Read the model definition and answer for the solid it produces. Units are mm, in the model's axes. A direction names the side the tool comes from. Coordinates: 2 decimals unless noted, no trailing zeros. Loops run counter-clockwise (first coordinate to the right, second up) from the corner with the lowest first, then second, coordinate; pieces in that order, holes last.
Q1. Section B-B (z = 3) is taken. Give the vertices of the cut face in (x, y), then the cut area to 3 significant figures.
Q2. Which of the six approach directions +Z, -Z, +X, -X, +Y, -Y give full straight-line access (tool end or side, diameter ignored) to faces 5 (the face through (6.35, 25, 7)), 6 (the face through (12.7, 25, 7)), 7 (the face through (9, 25, 10.16)), 8 (the face through (9, 26, 6.35)), 9 (the face through (-2.974, 5.098, -33.82))?
Q3. Section A-A (y = 33.5) is taken. Give the vertices of the cut face in (x, z).
Q4. Section D-D (z = -41) is taken. Give the vertices of the cut face in (x, y).
Q5. Straight lines are drawn through the part: line 1 (Y direction, x = 4, z = -32.5); line 2 (Y direction, x = -42, z = -5); line 3 (X direction, y = 42.5, z = 5). For each, find the intervals that lie inside material, in ascending order.
Q6. Flat-ended cylindrical pins translate along their axes: P1, Ø5, axis at x = 37.5, z = -27.5, coming from the +Y side; P2, Ø10, axis at y = 19.5, z = 1, coming from the +X side; P3, Ø2, axis at x = -2, y = 4.5, coming from the -Z side; P4, Ø2, axis at y = 40.5, z = -0.11, coming from the -X side. Find the tip coordinate at first contact, or state that the pin passes through.
Q7. The mould has two halves that part along Y. Classify faces 1 (the face through (9, 25, -10.16)), 2 (the face through (9, 26, -6.59)), 3 (the face through (1, 3.81, -32)), 4 (the face through (9, 38.079, 0)): pulls with the +Y half, pulls with the -Y half, needs draft (parallel to the pull), parting line crosses it, or undercut.
Q8. Section C-C (x = -2) is taken. Give the vertices of the cut face in (y, z), then the cut area to 3 significant figures.
from build123d import *

# Parameters (mm, degrees)
SKETCH1_R           = 50.8
BOSS_EXTRUDE1_DEPTH = 6.35
SKETCH2_W           = 6.35
SKETCH2_H           = 20.32
BOSS_EXTRUDE2_DEPTH = 38.1
SKETCH3_R           = 1.1
SKETCH3_W           = 12.939919869
SKETCH3_H           = 22.881654632
CUT_EXTRUDE1_DEPTH  = 12.7
CUT_EXTRUDE2_DEPTH  = 2.54


with BuildPart() as part:
    # Sketch1 → Boss-Extrude1 (new body)
    with BuildSketch(Plane(origin=(0, 0, 0), x_dir=(1, 0, 0), z_dir=(0, 1, 0))):
        Circle(SKETCH1_R)
    extrude(amount=BOSS_EXTRUDE1_DEPTH)

    # Sketch2 → Boss-Extrude2 (add)
    with BuildSketch(Plane(origin=(0, 6.35, 0), x_dir=(1, 0, 0), z_dir=(0, 1, 0))):
        with Locations((9.525, 0)):
            Rectangle(SKETCH2_W, SKETCH2_H)
    extrude(amount=BOSS_EXTRUDE2_DEPTH)

    # Sketch3 → Cut-Extrude1 (cut)
    with BuildSketch(Plane(origin=(6.35, 55.246794414, 64.642959957), x_dir=(0, 0, 1), z_dir=(-1, 0, 0))):
        with Locations((-64.750269074, -14.746794414)):
            Circle(SKETCH3_R)
        with Locations((-64.750269074, -42.546794414)):
            Circle(SKETCH3_R)
        with Locations((-64.762919892, -28.608275818)):
            Rectangle(SKETCH3_W, SKETCH3_H)
    extrude(amount=-CUT_EXTRUDE1_DEPTH, mode=Mode.SUBTRACT)

    # Sketch4 → Cut-Extrude2 (cut)
    with BuildSketch(Plane(origin=(0, 6.35, 0), x_dir=(1, 0, 0), z_dir=(0, 1, 0))):
        Polygon((-7.230978109, 23.634136505), (9.560420722, 23.634136505), (1.164721306, 43.725579037), align=None)
    extrude(amount=-CUT_EXTRUDE2_DEPTH, mode=Mode.SUBTRACT)


solid = part.part
Numbers:
1. outline: (-50.71, 0) - (50.71, 0) - (50.71, 6.35) - (12.7, 6.35) - (12.7, 15.2) - (6.35, 15.2) - (6.35, 6.35) - (-50.71, 6.35) - close; (6.35, 38.08) - (12.7, 38.08) - (12.7, 44.45) - (6.35, 44.45) - close
1. area: 741 mm2
2. face 5: +Z, -Z, -X, +Y
2. face 6: +Z, -Z, +X, +Y
2. face 7: +Z, +X, -X, +Y
2. face 8: +X, -X
2. face 9: +Y
3. outline: (6.35, -10.16) - (12.7, -10.16) - (12.7, -6.59) - (6.35, -6.59) - close; (6.35, 6.35) - (12.7, 6.35) - (12.7, 10.16) - (6.35, 10.16) - close
4. outline: (-29.99, 0) - (29.99, 0) - (29.99, 6.35) - (2.3, 6.35) - (2.3, 3.81) - (0.03, 3.81) - (0.03, 6.35) - (-29.99, 6.35) - close
5. line 1: y = 0 to 3.81
5. line 2: y = 0 to 6.35
5. line 3: x = 6.35 to 12.7
6. P1: stops at y = 6.35
6. P2: stops at x = 12.7
6. P3: stops at z = -50.79
6. P4: passes through
7. face 1: needs draft
7. face 2: undercut
7. face 3: pulls with the +Y half
7. face 4: undercut
8. outline: (0, -50.76) - (6.35, -50.76) - (6.35, -36.15) - (3.81, -36.15) - (3.81, -23.63) - (6.35, -23.63) - (6.35, 50.76) - (0, 50.76) - close
8. area: 613 mm2
